Autodesk Inventor part; units mm, degrees
ref_plane "YZ Plane" through (0, 0, 0) normal (1, 0, 0) x (0, 1, 0)
ref_plane "XZ Plane" through (0, 0, 0) normal (0, 1, 0) x (-1, 0, 0)
ref_plane "XY Plane" through (0, 0, 0) normal (0, 0, 1) x (1, 0, 0)
sketch "スケッチ1" plane through (0, 0, 0) normal (0, 1, 0) x (-1, 0, 0)
  circle A0 centre (0, 0) radius 7.5
  dimension "d0" = 15
extrude "押し出し1" add sketch "スケッチ1" along normal blind 1
sketch "スケッチ2" plane through (0, 1, 0) normal (0, 1, 0) x (1, 0, 0)
  circle A0 centre (0, 0) radius 7.5
  line L0 (0, 0) -> (-7.5, 0)
  line L1 (0, 0) -> (-1.3681, 3.7588)
  line L2 (-7.5, 0) -> (-6.4952, 3.75) construction
  line L3 (-6.4952, 3.75) -> (-1.3681, 3.7588) construction
  spline S0 degree 2 poles (-7.5, 0) (-6.4952, 3.75) (-1.3681, 3.7588) knots 1 1 1 2 2 2
  line L4 (-6.4952, 3.75) -> (-5.3033, 5.3033) construction
  line L5 (-5.3033, 5.3033) -> (-1.3681, 3.7588) construction
  spline S1 degree 2 poles (-6.4952, 3.75) (-5.3033, 5.3033) (-1.3681, 3.7588) knots 1 1 1 2 2 2
  line L6 (0, 0) -> (-5.3033, 5.3033)
  line L7 (-6.4952, 3.75) -> (0, 0)
  point P0 (-6.4952, 3.75)
  dimension "d5" = 70
  dimension "d14" = 4
  dimension "d18" = 25
  dimension "d19" = 15
extrude "押し出し2" add sketch "スケッチ2" along normal blind 3 contours A0 L7 S0 | S1 L6 S0 L7 | S1 S0 L6
pattern_circular "円形状パターン1" count 6 over 360 about axis through (0, 1, 0) along (0, 1, 0) of "押し出し2"
sketch "スケッチ4" plane through (0, 1, 0) normal (0, 1, 0) x (1, 0, 0)
  circle A0 centre (0, 0) radius 1
  dimension "d20" = 2
extrude "押し出し4" add sketch "スケッチ4" along normal blind 2 and the other way blind 2
fillet "フィレット1" radius 3 1 edges at (-1, 1, 0)
sketch "スケッチ5" plane through (0, 3, 0) normal (0, 1, 0) x (1, 0, 0)
  circle A0 centre (0, 0) radius 0.4
  dimension "d24" = 0.8
extrude "押し出し5" cut sketch "スケッチ5" against normal through all
fillet "フィレット2" radius 2 1 edges at (-1, 0, 0)
properties part number "Fan2"
Part model, mm, in its own coordinate system. Give positions to 0.01 mm unless a question says otherwise; leave off trailing zeros. Write each loop counter-clockwise with the first axis right and the second up, starting at its lowest first coordinate (ties: lowest second). Pieces come first, ordered by that corner, then holes. Notation, with made-up numbers: (0, 8.5) -> (18, 8.5) arc R21 ccw to (18, 34.5) -> close; hole circle Ø5 at (0, 75.5). An arc over 180 degrees is marked (long way). Put each result on its own line as item: value. Start each with the question number.
Item 1: Pin check, flat tips, straight feed: pin 1 Ø1 at (x, y) = (2.5, 2.5) entering from +Z; pin 2 Ø1 at (x, z) = (4.5, -3) entering from -Y; pin 3 Ø4.5 at (x, z) = (2.5, 2.5) entering from -Y; pin 4 Ø0.6 at (x, z) = (0, 0) entering from +Y. Stop position of each tip, or through.
Item 2: Cut at A-A (y = 1.7). State how many separate pieces and enclosed holes the cut face has, then the cut area to 3 significant figures.
Item 3: Pull direction Z, two halves, no side cores. Call faces 1 (the face through (-3, 1, -3)), 2 (the face through (0, 0, -3)): pulls with the +Z half, pulls with the -Z half, needs draft (parallel to the pull), parting line crosses it, or undercut.
Item 4: Cut at B-B (y = -0.2). List the corners of the cut face in (x, z), then the cut area to 3 significant figures.
Item 5: Wall check: L1, parallel to X at y = 2.4, z = 1; L2, parallel to X at y = 0.25, z = 0; L3, parallel to Z at x = 0, y = 1.95. Give the ranges that are in metal, low to high. Write a range as [from, to].
Answer list:
1. pin 1: stops at z = 7.23
1. pin 2: stops at y = 0
1. pin 3: stops at y = -0.62
1. pin 4: passes through
2. separate pieces: 7
2. enclosed holes: 1
2. area: 50.0 mm2
3. face 1: undercut
3. face 2: needs draft
4. outline: circle Ø3.72 at (0, 0); hole circle Ø0.8 at (0, 0)
4. area: 10.4 mm2
5. L1: x = [-5.72, -4.74], [-0.82, 0.82], [7.13, 7.43]
5. L2: x = [-7.5, -0.4], [0.4, 7.5]
5. L3: z = [-7.5, -5.97], [-1.64, -0.4], [0.4, 1.64], [5.97, 7.5]
